Check sheet for the drawn part. Datum: minimum x, y, z corner. Units: mm. A direction names the side the tool comes from. Give positions to 0.01 mm unless a question says otherwise; leave off trailing zeros. Order: outer loops, then holes, each group sorted by start corner. A loop starts at its lowest first (then second) coordinate and runs counter-clockwise, first axis right, second up.
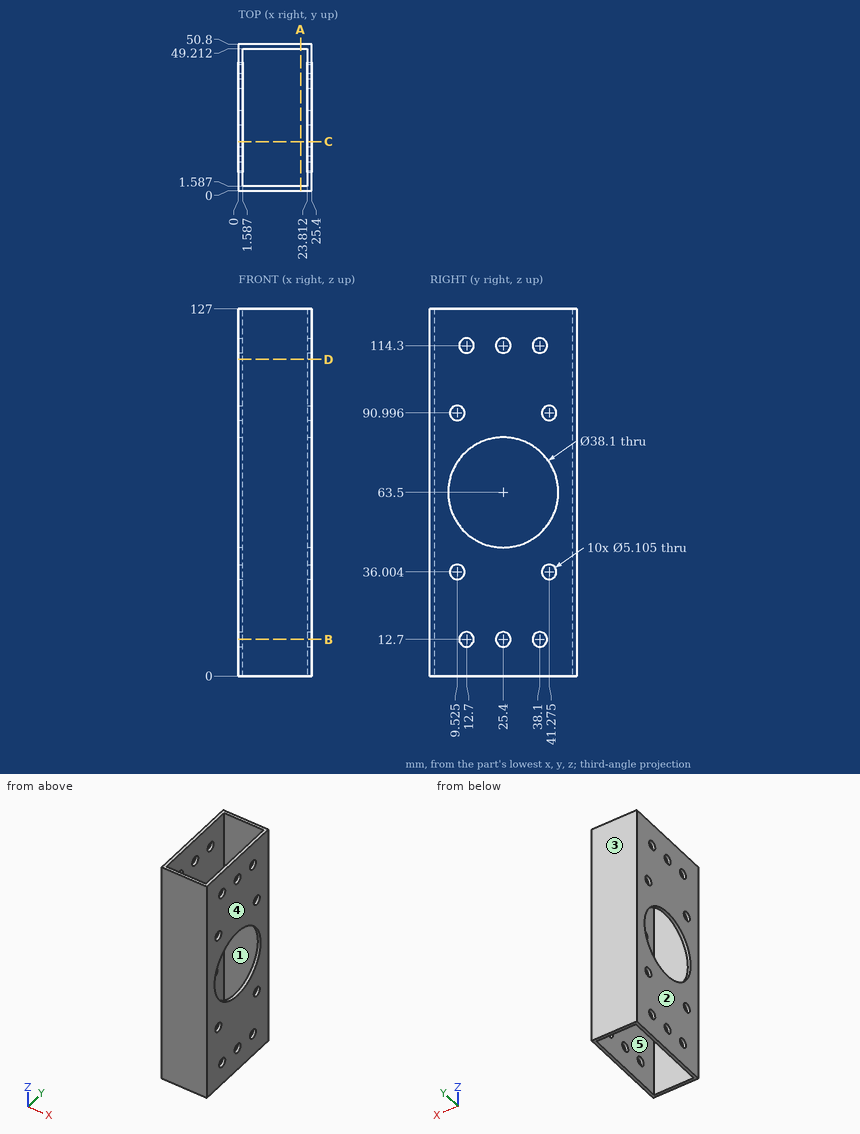
(1) Section check C-C, the plane y = 17. Enter the section's corners in (x, z).
Solved:
outline: (0, 0) - (1.59, 0) - (1.59, 46.4) - (0, 46.4) - close; (0, 80.6) - (1.59, 80.6) - (1.59, 127) - (0, 127) - close; (23.81, 0) - (25.4, 0) - (25.4, 46.4) - (23.81, 46.4) - close; (23.81, 80.6) - (25.4, 80.6) - (25.4, 127) - (23.81, 127) - close
(2) Section check B-B, the plane z = 12.7. Give the number of separate pieces and of enclosed holes in the cut face, then the cut area to 3 significant figures.
Solved:
separate pieces: 6
enclosed holes: 0
area: 183 mm2
(3) Release check for a two-part mould opening along X. For the marked faces 3, 4 and 5 record: pulls with the +X half, pulls with the -X half, needs draft (parallel to the pull), parting line crosses it, or undercut.
Solved:
face 3: needs draft
face 4: pulls with the +X half
face 5: undercut
(4) Section check A-A, the plane x = 21.5. Enter the section's corners in (y, z).
Solved:
outline: (0, 0) - (1.59, 0) - (1.59, 127) - (0, 127) - close; (49.21, 0) - (50.8, 0) - (50.8, 127) - (49.21, 127) - close
(5) Go/stop test with a flat-tipped pin: pin 1 (6 mm diameter, centred on y = 12.7, z = 12.7, fed in from -X). Record where the tip stops, or that it passes through.
Solved:
pin 1: stops at x = 0
(6) Set-up check for the marked faces 1 and 2: record each of +Z, -Z, +X, -X, +Y, -Y from which the full face is reachable in a straight line by a thin tool's end or side.
Solved:
face 1: +Z, -Z
face 2: +Z, -Z, -X, +Y, -Y
(7) Scan lines: line 1 (Y direction, x = 24.65, z = 12.7); line 2 (X direction, y = 8, z = 115); line 3 (Y direction, x = 13.25, z = 93.5). Record each from-to range of solid material in increasing order.
Solved:
line 1: y = 0 to 10.15, 15.25 to 22.85, 27.95 to 35.55, 40.65 to 50.8
line 2: x = 0 to 1.59, 23.81 to 25.4
line 3: y = 0 to 1.59, 49.21 to 50.8
(8) Section check D-D, the plane z = 109.5. Enter the section's corners in (x, y).
Solved:
outline: (0, 0) - (25.4, 0) - (25.4, 50.8) - (0, 50.8) - close; hole (1.59, 1.59) - (23.81, 1.59) - (23.81, 49.21) - (1.59, 49.21) - close
